```python
from build123d import *

# Parameters (mm, degrees)
FILLET2_R = 0.5


with BuildPart() as part:
    # Sketch1 → Revolve1 (revolve)
    with BuildSketch(Plane(origin=(0, 0, 0), x_dir=(0, 0, -1), z_dir=(1, 0, 0)), mode=Mode.PRIVATE) as revolve1_sk:
        Polygon((13.7, 30.5), (13.7, 29.597484089), (80.7, 29.597484089), (80.7, 11.585161601), (88.164497018, 11.585161601), (88.164497018, 4), (90.391404279, 4), (90.391404279, 0), (-36.308595721, 0), (-36.308595721, 4), (5.413824797, 4), (5.413824797, 5.652900668), (0, 5.652900668), (0, 30.5), align=None)
    revolve(revolve1_sk.sketch.rotate(Axis((0, 0, 36.308595721), (0, 0, -1)), 90), axis=Axis((0, 0, 36.308595721), (0, 0, -1)))

    # Fillet2
    fillet2_edges = [part.edges().sort_by_distance(p)[0] for p in [
        (-4, 0, 36.308595721),
        (-4, 0, -90.391404279),
        (-29.597484089, 0, -80.7),
        (-30.5, 0, 0),
    ]]
    fillet(fillet2_edges, radius=FILLET2_R)


solid = part.part
```
Check sheet for the modelled part. Datum: model origin and axes. Units: mm. A direction names the side the tool comes from. Coordinates: 2 decimals unless noted, no trailing zeros. Loops run counter-clockwise (first coordinate to the right, second up) from the corner with the lowest first, then second, coordinate; pieces in that order, holes last.
1) Gauge pin test, flat ends, axial feed: pin 1 (10 mm diameter, centred on x = -9.5, y = -10, fed in from +Z); pin 2 (1 mm diameter, centred on y = 4.5, z = -41.5, fed in from +X); pin 3 (3 mm diameter, centred on x = 21.5, z = -18, fed in from -Y). Record the tip position at first contact, or that the pin passes through.
2) Material ranges on probe 1 along Y at (x, z) = (0, -3.05); probe 2 along Z at (x, y) = (-6.5, 27); probe 3 along Z at (x, y) = (3, 7), recorded low to high.
3) Sectioned sample at C-C (z = -83). Record the boundary of the cut face in (x, y), and give its area (3 significant figures).
4) Access from +Z, -Z, +X, -X, +Y, -Y to the whole of each face (thin tool, end or side, straight path). Record for faces 4 (the face through (-2, 4, -5.414)), 5 (the face through (0, 5, -88.164)), 6 (the face through (0, 0, -90.391)).
5) Sectioned sample at D-D (z = -55). Record the boundary of the cut face in (x, y).
6) Release check for a two-part mould opening along X. For faces 1 (the face through (-8.54, -7.83, -84.48)), 2 (the face through (-4.166, -3.82, -2.669)), 3 (the face through (-2, -30, -13.7)) record: released by +X, released by -X, zero draft, split by the parting line, or undercut.
Check sheet entries:
1. pin 1: stops at z = 0
1. pin 2: stops at x = 29.33
1. pin 3: stops at y = -21.82
2. probe 1: y = -30.5 to -5.65, -4 to 4, 5.65 to 30.5
2. probe 2: z = -80.7 to 0
2. probe 3: z = -88.16 to 0
3. outline: circle Ø23.17 at (0, 0)
3. area: 422 mm2
4. face 4: +Z
4. face 5: -Z
4. face 6: -Z, +X, -X, +Y, -Y
5. outline: circle Ø59.19 at (0, 0)
6. face 1: split by the parting line
6. face 2: undercut
6. face 3: zero draft
